Can you work these out from the model? Positions are in its coordinate system, mm. Face numbers are marked on the shaded views. A direction names the side the tool comes from. Coordinates: 2 decimals unless noted, no trailing zeros. Order: outer loops, then holes, each group sorted by start corner. A loop starts at its lowest first (then second) coordinate and runs counter-clockwise, first axis right, second up. Notation, with made-up numbers: (37.5, 38) -> (61.5, 38) arc R10 cw to (61.5, 43) -> close; hole circle Ø8 at (67, 24.5). An arc over 180 degrees is marked (long way). Answer in a Markdown table with one row per item. Add a question column.
1. Imagine slicing it at A-A on x = 0. Write out the boundary of the cut face in (y, z).
2. On a 3-axis mill with a long thin cutter (end or side, diameter ignored), from which of +Z, -Z, +X, -X, +Y, -Y can I reach the whole of each face in a straight line? I mean the marked faces 1 and 2. Say none if no direction works.
3. Will these pins go through, and if not, where does the flat tip stop? pin 1 (3 mm diameter, centred on y = -5.5, z = -16.5, fed in from -X); pin 2 (12 mm diameter, centred on x = -7.5, y = 7, fed in from -Z); pin 3 (10 mm diameter, centred on y = 1.5, z = -17, fed in from +X); pin 4 (2 mm diameter, centred on x = -2.5, z = -19, fed in from -Y).
4. Imagine slicing it at C-C on x = 7. Write out the boundary of the cut face in (y, z).
5. If I drill on line 1 along Y through (x, z) = (0, 3.3); line 2 along Z through (x, y) = (5.5, -8.25); line 3 along Y through (x, z) = (-7, 1.8), over which ranges is the centre line in solid material (lowest first)? Write a range as [from, to].
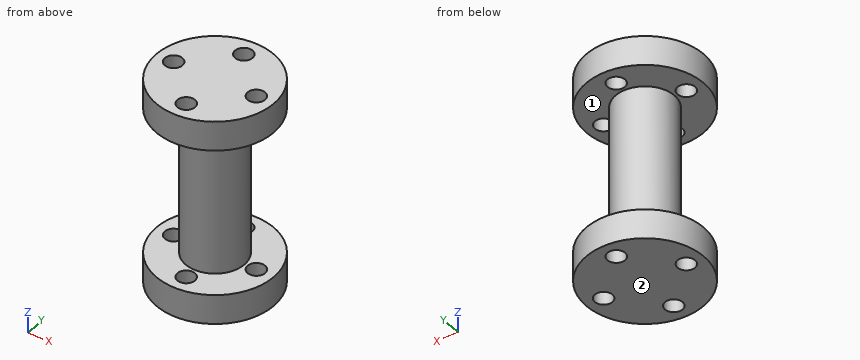
Autodesk Fusion 360 part; units mm, degrees
sketch "Sketch1" plane through (0, 0, 0) normal (0, 0, 1) x (1, 0, 0)
  circle A0 centre (0, 0) radius 7 construction
  circle A1 centre (-7, 0) radius 1.5
  circle A2 centre (0, 7) radius 1.5
  circle A3 centre (7, 0) radius 1.5
  circle A4 centre (0, -7) radius 1.5
  circle A5 centre (0, 0) radius 10
  circle A6 centre (0, 0) radius 5
  dimension "d5" = 360
  dimension "d7" = 14
  dimension "d8" = 3
  dimension "d11" = 20
  dimension "d15" = 10
extrude "Extrude1" add sketch "Sketch1" along normal blind 5 contours A5 | A6
extrude "Extrude2" add sketch "Sketch1" against normal blind 30 contours A6
sketch "Sketch3" plane through (0, 0, -30) normal (0, 0, -1) x (1, 0, 0)
  circle A0 centre (0, 0) radius 5
  circle A1 centre (0, 7) radius 1.5
  circle A2 centre (0, 0) radius 5
  circle A3 centre (0, 0) radius 7 construction
  circle A4 centre (-7, 0) radius 1.5
  circle A5 centre (0, -7) radius 1.5
  circle A6 centre (7, 0) radius 1.5
  circle A7 centre (0, 0) radius 10
  dimension "d20" = 360
  dimension "d21" = 14
  dimension "d22" = 3
  dimension "d23" = 20
  dimension "d24" = 10
extrude "Extrude4" add sketch "Sketch3" against normal blind 5
equation "outer_radius = 20 mm"
equation "radius_thickness = 5 mm"
equation "d11 = outer_radius"
equation "d12 = radius_thickness"
equation "inner_radius = 10 mm"
equation "d15 = inner_radius"
equation "tot_height = 35 mm"
equation "d23 = outer_radius"
equation "d24 = inner_radius"
Answers follow:
| question | item | result |
|---|---|---|
| 1 | outline | (-10, -30) -> (-8.5, -30) -> (-8.5, -25) -> (-10, -25) -> close; (-10, 0) -> (-8.5, 0) -> (-8.5, 5) -> (-10, 5) -> close; (-5.5, -30) -> (5.5, -30) -> (5.5, -25) -> (5, -25) -> (5, 0) -> (5.5, 0) -> (5.5, 5) -> (-5.5, 5) -> (-5.5, 0) -> (-5, 0) -> (-5, -25) -> (-5.5, -25) -> close; (8.5, -30) -> (10, -30) -> (10, -25) -> (8.5, -25) -> close; (8.5, 0) -> (10, 0) -> (10, 5) -> (8.5, 5) -> close |
| 2 | face 1 | none |
| 2 | face 2 | -Z, +X, -X, +Y, -Y |
| 3 | pin 1 | stops at x = -3 |
| 3 | pin 2 | stops at z = -30 |
| 3 | pin 3 | stops at x = 5 |
| 3 | pin 4 | stops at y = -4.77 |
| 4 | outline | (-7.14, -30) -> (-1.5, -30) -> (-1.5, -25) -> (-7.14, -25) -> close; (-7.14, 0) -> (-1.5, 0) -> (-1.5, 5) -> (-7.14, 5) -> close; (1.5, -30) -> (7.14, -30) -> (7.14, -25) -> (1.5, -25) -> close; (1.5, 0) -> (7.14, 0) -> (7.14, 5) -> (1.5, 5) -> close |
| 5 | line 1 | y = [-10, -8.5], [-5.5, 5.5], [8.5, 10] |
| 5 | line 2 | z = [-30, -25], [0, 5] |
| 5 | line 3 | y = [-7.14, -1.5], [1.5, 7.14] |
